Read the model definition and answer for the solid it produces. Units are mm, in the model's axes. A direction names the side the tool comes from. Give positions to 0.01 mm unless a question says otherwise; leave off trailing zeros. Write each loop counter-clockwise with the first axis right and the second up, starting at its lowest first coordinate (ties: lowest second). Pieces come first, ordered by that corner, then holes.
```python
from build123d import *

# Parameters (mm, degrees)
ESQUISSE1_R        = 1.6
ESQUISSE1_R_2      = 2.25
ESQUISSE1_W        = 20
ESQUISSE1_H        = 20
BOSS_EXTRU_1_DEPTH = 5


with BuildPart() as part:
    # Esquisse1 → Boss.-Extru.1 (new body)
    with BuildSketch(Plane.XY):
        with BuildLine():
            Line((0, 0), (150, 0))
            Line((150, 0), (150, -100))
            ThreePointArc((150, -100), (144.142135624, -114.142135624), (130, -120))
            Line((130, -120), (20, -120))
            ThreePointArc((20, -120), (5.857864376, -114.142135624), (0, -100))
            Line((0, -100), (0, 0))
        make_face()
        with Locations((52, -61)):
            Circle(ESQUISSE1_R, mode=Mode.SUBTRACT)
        with Locations((110, -61)):
            Circle(ESQUISSE1_R, mode=Mode.SUBTRACT)
        with Locations((110, -110)):
            Circle(ESQUISSE1_R, mode=Mode.SUBTRACT)
        with Locations((52, -110)):
            Circle(ESQUISSE1_R, mode=Mode.SUBTRACT)
        with Locations((8.5, -31)):
            Circle(ESQUISSE1_R_2, mode=Mode.SUBTRACT)
        with Locations((141.5, -31)):
            Circle(ESQUISSE1_R_2, mode=Mode.SUBTRACT)
        with Locations((25, -10)):
            Circle(ESQUISSE1_R_2, mode=Mode.SUBTRACT)
        with Locations((125, -10)):
            Circle(ESQUISSE1_R_2, mode=Mode.SUBTRACT)
        with Locations((96, -30)):
            Circle(ESQUISSE1_R_2, mode=Mode.SUBTRACT)
        with Locations((54, -30)):
            Circle(ESQUISSE1_R_2, mode=Mode.SUBTRACT)
        with Locations((75, -10)):
            Circle(ESQUISSE1_R_2, mode=Mode.SUBTRACT)
        with Locations((75, -30)):
            Rectangle(ESQUISSE1_W, ESQUISSE1_H, mode=Mode.SUBTRACT)
    extrude(amount=BOSS_EXTRU_1_DEPTH)


solid = part.part
```
Item 1: Section D-D (x = 110) is taken. Write down the section's boundary in (y, z), and give its area (3 significant figures).
Result set:
outline: (-120, 0) - (-111.6, 0) - (-111.6, 5) - (-120, 5) - close; (-108.4, 0) - (-62.6, 0) - (-62.6, 5) - (-108.4, 5) - close; (-59.4, 0) - (0, 0) - (0, 5) - (-59.4, 5) - close
area: 568 mm2
Item 2: Each of these flat-tipped pins is pushed along its axis until it touches: pin 1 Ø5 at (x, y) = (54, -30) entering from +Z; pin 2 Ø2.5 at (x, y) = (52, -61) entering from +Z. Where does it stop, or does it pass through?
Result set:
pin 1: stops at z = 5
pin 2: passes through
Item 3: Section A-A (y = -61) is taken. Write down the section's boundary in (x, z).
Result set:
outline: (0, 0) - (50.4, 0) - (50.4, 5) - (0, 5) - close; (53.6, 0) - (108.4, 0) - (108.4, 5) - (53.6, 5) - close; (111.6, 0) - (150, 0) - (150, 5) - (111.6, 5) - close
Item 4: Which of the six approach directions +Z, -Z, +X, -X, +Y, -Y give full straight-line access (tool end or side, diameter ignored) to faces 1 (the flat face through (0, -51, 2)), 2 (the flat face through (85, -30, 2))?
Result set:
face 1: +Z, -Z, -X, +Y, -Y
face 2: +Z, -Z
Item 5: Section B-B (x = 70.5) is taken. Write down the section's boundary in (y, z).
Result set:
outline: (-120, 0) - (-40, 0) - (-40, 5) - (-120, 5) - close; (-20, 0) - (0, 0) - (0, 5) - (-20, 5) - close
Item 6: Section C-C (z = 3.7) is taken. Give the number of separate pieces and of enclosed holes in the cut face, and give its area (3 significant figures).
Result set:
separate pieces: 1
enclosed holes: 12
area: 17,300 mm2
Item 7: Determine the mould class of faces 3 (the cylindrical face through (6.014, -114.297, 2.465)), 4 (the flat face through (74, 0, 2)), 5 (the cylindrical face through (51.752, -29.901, 2.465)), 6 (the flat face through (150, -49, 2)) for opening direction Y: pulls with the +Y half, pulls with the -Y half, needs draft (parallel to the pull), parting line crosses it, or undercut.
Result set:
face 3: pulls with the -Y half
face 4: pulls with the +Y half
face 5: undercut
face 6: needs draft
Item 8: Find the intervals of material crossed by line 1 along Y through (x, z) = (52, 2.15); line 2 along Y through (x, z) = (96, 3.6); line 3 along Y through (x, z) = (51.5, 1.5), in increasing order.
Result set:
line 1: y = -120 to -111.6, -108.4 to -62.6, -59.4 to -31.03, -28.97 to 0
line 2: y = -120 to -32.25, -27.75 to 0
line 3: y = -120 to -111.52, -108.48 to -62.52, -59.48 to 0
